The listing builds one solid part. Answer for the finished solid, in the listing's coordinates (mm). A direction names the side the tool comes from. Round coordinates to 2 decimals unless told otherwise and drop trailing zeros. Order: outer loops, then holes, each group sorted by start corner. A loop starts at its lowest first (then second) coordinate and runs counter-clockwise, first axis right, second up. Notation, with made-up numbers: (77.25, 27.25) - (117.25, 27.25) arc R23 ccw to (117.25, 54.25) - close; hole circle Ø5 at (89.25, 34.25). An arc over 180 degrees is marked (long way). Write item = value, one per line.
from build123d import *

# Parameters (mm, degrees)
EXTRUDE_1_DEPTH     = 50
SKETCH_2_W          = 15
SKETCH_2_H          = 1.5
CUT_EXTRUDE_1_DEPTH = 0.2
SKETCH_5_W          = 15
SKETCH_5_H          = 1.5
EXTRUDE_2_DEPTH     = 0.15
EXTRUDE_4_DEPTH     = 5
SKETCH_9_W          = 7
SKETCH_9_H          = 10
EXTRUDE_5_DEPTH     = 12
FILLET_2_R          = 5
SKETCH_10_R         = 1.5
CUT_EXTRUDE_3_DEPTH = 57.808890149
CUT_EXTRUDE_4_DEPTH = 15


with BuildPart() as part:
    # 草图1 → 凸台-拉伸1 (new body)
    with BuildSketch(Plane(origin=(0, 0, 0), x_dir=(1, 0, 0), z_dir=(0, 1, 0))):
        with BuildLine():
            Line((-11, 3.3), (11, 3.3))
            ThreePointArc((11, 3.3), (14.3, 0), (11, -3.3))
            Line((11, -3.3), (-11, -3.3))
            ThreePointArc((-11, -3.3), (-14.3, 0), (-11, 3.3))
        make_face()
    extrude(amount=EXTRUDE_1_DEPTH)

    # 草图2 → 切除-拉伸1 (cut)
    with BuildSketch(Plane(origin=(0, 0, -3.3), x_dir=(-1, 0, 0), z_dir=(0, 0, -1))):
        with Locations((0, 37.5)):
            Rectangle(SKETCH_2_W, SKETCH_2_H)
        with Locations((0, 12.5)):
            Rectangle(SKETCH_2_W, SKETCH_2_H)
        with Locations((0, 25)):
            Rectangle(SKETCH_2_W, SKETCH_2_H)
    extrude(amount=-CUT_EXTRUDE_1_DEPTH, mode=Mode.SUBTRACT)

    # 草图5 → 凸台-拉伸2 (add)
    with BuildSketch(Plane(origin=(0, 0, -3.3), x_dir=(-1, 0, 0), z_dir=(0, 0, -1))):
        with Locations((0, 49.25)):
            Rectangle(SKETCH_5_W, SKETCH_5_H)
    extrude(amount=EXTRUDE_2_DEPTH)

    # 草图8 → 凸台-拉伸4 (add)
    with BuildSketch(Plane.XZ):
        with BuildLine():
            Line((-11, -5), (11, -5))
            ThreePointArc((11, -5), (16, 0), (11, 5))
            Line((11, 5), (-11, 5))
            ThreePointArc((-11, 5), (-16, 0), (-11, -5))
        make_face()
    extrude(amount=EXTRUDE_4_DEPTH)

    # 草图9 → 凸台-拉伸5 (add)
    with BuildSketch(Plane.XZ.offset(5)):
        with Locations((-7, 0)):
            Rectangle(SKETCH_9_W, SKETCH_9_H)
        with Locations((7, 0)):
            Rectangle(SKETCH_9_W, SKETCH_9_H)
    extrude(amount=EXTRUDE_5_DEPTH)

    # 圆角2
    fillet_2_edges = [part.edges().sort_by_distance(p)[0] for p in [
        (7, -17, 5),
        (7, -17, -5),
        (-7, -17, 5),
        (-7, -17, -5),
    ]]
    fillet(fillet_2_edges, radius=FILLET_2_R - 0.0001)  # a hair under: the kernel refuses the full size

    # 草图10 → 切除-拉伸3 (cut, through all)
    with BuildSketch(Plane(origin=(10.5, 0, 0), x_dir=(0, 0, -1), z_dir=(1, 0, 0))):
        with Locations((0, -12)):
            Circle(SKETCH_10_R)
    extrude(amount=-CUT_EXTRUDE_3_DEPTH, mode=Mode.SUBTRACT)

    # 草图11 → 切除-拉伸4 (cut)
    with BuildSketch(Plane(origin=(-7.5, 0, 0), x_dir=(0, 0, -1), z_dir=(1, 0, 0))):
        with BuildLine():
            Line((3.3, 38.45), (3.3, 38.25))
            Line((3.3, 38.25), (3.1, 38.25))
            ThreePointArc((3.1, 38.25), (3.158578644, 38.391421356), (3.3, 38.45))
        make_face()
        with BuildLine():
            Line((3.3, 36.75), (3.3, 36.55))
            ThreePointArc((3.3, 36.55), (3.158578644, 36.608578644), (3.1, 36.75))
            Line((3.1, 36.75), (3.3, 36.75))
        make_face()
        with BuildLine():
            Line((3.3, 25.95), (3.3, 25.75))
            Line((3.3, 25.75), (3.1, 25.75))
            ThreePointArc((3.1, 25.75), (3.158578644, 25.891421356), (3.3, 25.95))
        make_face()
        with BuildLine():
            Line((3.3, 13.45), (3.3, 13.25))
            Line((3.3, 13.25), (3.1, 13.25))
            ThreePointArc((3.1, 13.25), (3.158578644, 13.391421356), (3.3, 13.45))
        make_face()
        with BuildLine():
            Line((3.3, 24.25), (3.3, 24.05))
            ThreePointArc((3.3, 24.05), (3.158578644, 24.108578644), (3.1, 24.25))
            Line((3.1, 24.25), (3.3, 24.25))
        make_face()
        with BuildLine():
            Line((3.3, 11.75), (3.3, 11.55))
            ThreePointArc((3.3, 11.55), (3.158578644, 11.608578644), (3.1, 11.75))
            Line((3.1, 11.75), (3.3, 11.75))
        make_face()
    extrude(amount=CUT_EXTRUDE_4_DEPTH, mode=Mode.SUBTRACT)


solid = part.part
Q1. Find the intervals of material crossed by line 1 (Y direction, x = -8.5, z = 0); line 2 (Y direction, x = 12.5, z = -3.5); line 3 (Z direction, x = -0.5, y = 6.5), in increasing order. Write a range as from..to.
Model answer:
line_1 = -17..-13.5, -10.5..50
line_2 = -5..0
line_3 = -3.3..3.3
Q2. Section D-D on y = 39.5 is taken. Determine the outline of the cut face in (x, z).
Model answer:
outline = (-11, -3.3) - (11, -3.3) arc R3.3 ccw to (11, 3.3) - (-11, 3.3) arc R3.3 ccw to start
Q3. Section B-B on x = 1.5 is taken. Determine the outline of the cut face in (y, z), then the cut area to 3 significant figures.
Model answer:
outline = (-5, -5) - (0, -5) - (0, -3.3) - (11.55, -3.3) arc R0.2 cw to (11.75, -3.1) - (13.25, -3.1) arc R0.2 cw to (13.45, -3.3) - (24.05, -3.3) arc R0.2 cw to (24.25, -3.1) - (25.75, -3.1) arc R0.2 cw to (25.95, -3.3) - (36.55, -3.3) arc R0.2 cw to (36.75, -3.1) - (38.25, -3.1) arc R0.2 cw to (38.45, -3.3) - (48.5, -3.3) - (48.5, -3.45) - (50, -3.45) - (50, 3.3) - (0, 3.3) - (0, 5) - (-5, 5) - close
area = 379 mm^2
Q4. Determine the mould class of faces 1 (the face through (-6.951, -13.464, 0.325)), 2 (the face through (7, -15, 4)), 3 (the face through (3.5, -10, 0)) for opening direction Z: released by +Z, released by -Z, zero draft, split by the parting line, or undercut.
Model answer:
face_1 = undercut
face_2 = released by +Z
face_3 = zero draft
Q5. Flat-ended cylindrical pins translate along their axes: P1, Ø12, axis at x = -8.5, y = 30, coming from the +Z side; P2, Ø0.8, axis at x = -1, y = 25, coming from the -Z side; P3, Ø3.5, axis at x = -1, z = -1.5, coming from the -Y side. Find the tip coordinate at first contact, or state that the pin passes through.
Model answer:
P1 = 3.3
P2 = -3.1
P3 = -5
Q6. Section C-C on z = 4.25 is taken. Determine the outline of the cut face in (x, y).
Model answer:
outline = (-13.63, -5) - (-10.5, -5) - (-10.5, -14.63) - (-3.5, -14.63) - (-3.5, -5) - (3.5, -5) - (3.5, -14.63) - (10.5, -14.63) - (10.5, -5) - (13.63, -5) - (13.63, 0) - (-13.63, 0) - close
Q7. For faces 4 (the face through (0, 38, -3.1)), 5 (the face through (-10.5, -10, 0)), 6 (the face through (0, 49, -3.45)), determine the directions among +Z, -Z, +X, -X, +Y, -Y from which every point of the face is accessible in a straight line to the end or side of a thin tool.
Model answer:
face_4 = -Z
face_5 = +Z, -Z, -X, -Y
face_6 = -Z, +X, -X, +Y
